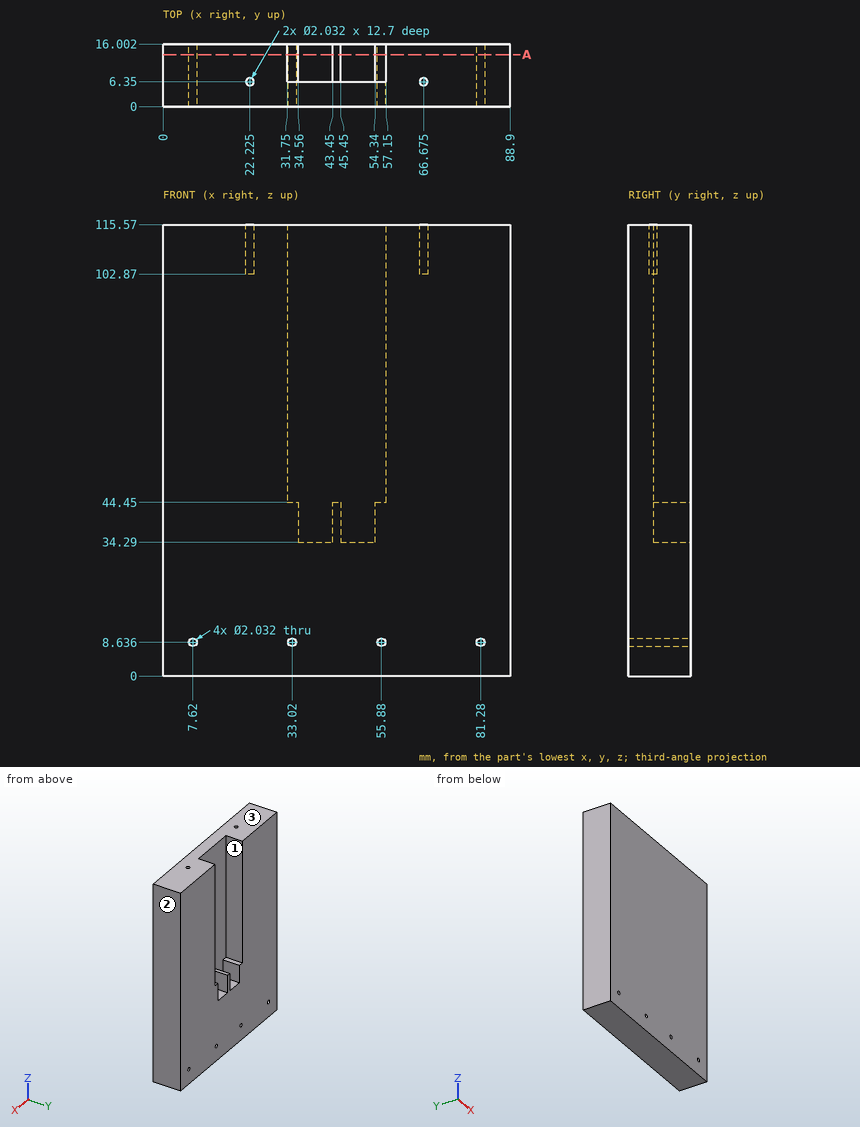
Design review of the part shown in the three views and the two pictorial views. Dimensions are in mm from the part's minimum x, y and z. Give positions to 0.01 mm unless a question says otherwise; leave off trailing zeros. Loops run counter-clockwise (first coordinate to the right, second up) from the corner with the lowest first, then second, coordinate; pieces in that order, holes last. Notation, with made-up numbers: M 63.5,75 L 73.5,75 A30 cw 73.5,103 Z; hole C -6,89.5 d1. An arc over 180 degrees is marked long. Write item = value, one per line.
Q1. We need section A-A (y = 13.25). Give the boundary of the cut face in (x, z), plus the area to 3 significant figures.
Output values:
outline = M 0,0 L 88.9,0 L 88.9,115.57 L 57.15,115.57 L 57.15,44.45 L 54.34,44.45 L 54.34,34.29 L 45.45,34.29 L 45.45,44.45 L 43.45,44.45 L 43.45,34.29 L 34.56,34.29 L 34.56,44.45 L 31.75,44.45 L 31.75,115.57 L 0,115.57 Z; hole C 7.62,8.64 d2.03; hole C 33.02,8.64 d2.03; hole C 55.88,8.64 d2.03; hole C 81.28,8.64 d2.03
area = 8,270 mm^2
Q2. Insertion check: pin 1 (0.6 mm diameter, centred on x = 22.5, y = 6.5, fed in from +Z); pin 2 (1.8 mm diameter, centred on x = 33.02, z = 8.636, fed in from -Y); pin 3 (4.5 mm diameter, centred on x = 50, y = 13.5, fed in from +Z); pin 4 (1.4 mm diameter, centred on x = 33, y = 10.5, fed in from +Z). Each pin has a flat end and moves straight along its axis. Give the tip position at first contact, or say it passes through.
Output values:
pin_1 = 102.87
pin_2 = through
pin_3 = 34.29
pin_4 = 44.45
Q3. Draft analysis for pull direction X (two halves, no side actions). For the marked faces 1, 2 and 3, state which applies: +X half, -X half, draft (parallel to the pull), parting line (faces both ways), or undercut.
Output values:
face_1 = undercut
face_2 = +X half
face_3 = draft
Q4. To check wall thickness, follow line 1 (Z direction, x = 33.02, y = 5); line 2 (X direction, y = 12, z = 53.5); line 3 (Z direction, x = 49, y = 10). State the ranges of each line that lie inside material, in increasing order. Write a range as [from, to].
Output values:
line_1 = [0, 7.62], [9.65, 115.57]
line_2 = [0, 31.75], [57.15, 88.9]
line_3 = [0, 34.29]
